Build history of the part. All positions in model axes, mm. Face numbers are marked on the shaded views. A direction names the side the tool comes from. Coordinates: 2 decimals unless noted, no trailing zeros. Loops run counter-clockwise (first coordinate to the right, second up) from the corner with the lowest first, then second, coordinate; pieces in that order, holes last.
Item 1: Cut at D-D (z = 3.5). List the corners of the cut face in (x, y), and give its area (3 significant figures).
Item 2: Cut at C-C (y = 13.5). List the corners of the cut face in (x, z).
Item 3: Flat gauge pins, fed straight in: pin 1 (12 mm diameter, centred on x = 25.5, y = 21.5, fed in from +Z); pin 2 (2.5 mm diameter, centred on y = 41.5, z = 9, fed in from +X); pin 3 (8 mm diameter, centred on y = 2.5, z = 14, fed in from -X). Where does each tip first touch, or does it go through?
Item 4: Cut at A-A (x = 30). List the corners of the cut face in (y, z).
Item 5: Drill centre lines: line 1 along Y through (x, z) = (53.5, 1.3); line 2 along X through (y, z) = (39.15, 12.5); line 3 along X through (y, z) = (34.5, 3.5). Where is each one in solid material? Low to high.
Item 6: Cut at B-B (z = 7). List the corners of the cut face in (x, y), and give its area (3 significant figures).
Item 7: 3-axis set-ups, long thin cutter, end or side, ignore diameter. For the marked faces 1, 2 and 3: which of +Z, -Z, +X, -X, +Y, -Y reach the whole face in a straight line?
Item 8: Mould opens along Y. For the marked faces 4, 5 and 6 say: released by +Y, released by -Y, zero draft, split by the parting line, or undercut.
Autodesk Inventor part; units mm, degrees
ref_plane "YZ Plane" through (0, 0, 0) normal (1, 0, 0) x (0, 1, 0)
ref_plane "XZ Plane" through (0, 0, 0) normal (0, 1, 0) x (-1, 0, 0)
ref_plane "XY Plane" through (0, 0, 0) normal (0, 0, 1) x (1, 0, 0)
sketch "Эскиз1" plane through (0, 0, 0) normal (0, 0, 1) x (1, 0, 0)
  arc A0 (50, 23.4174) -> (30, 23.4174) centre (40, 28) ccw
  line L0 (0, 37.25) -> (5.75, 43)
  line L1 (0, 0) -> (0, 37.25)
  line L2 (80, 0) -> (0, 0)
  line L3 (80, 0) -> (80, 37.25)
  line L4 (74.25, 43) -> (80, 37.25)
  line L5 (5.75, 43) -> (74.25, 43)
  circle A1 centre (40, 28) radius 2
  arc A2 (2.9, 3.4608) -> (7.1, 3.4608) centre (5, 3.4608) ccw
  line L6 (2.9, 3.4608) -> (2.9, 36.5392)
  arc A3 (7.1, 36.5392) -> (2.9, 36.5392) centre (5, 36.5392) ccw
  line L7 (7.1, 36.5392) -> (7.1, 3.4608)
  arc A4 (77.1, 36.5392) -> (72.9, 36.5392) centre (75, 36.5392) ccw
  line L8 (77.1, 36.5392) -> (77.1, 3.4608)
  arc A5 (72.9, 3.4608) -> (77.1, 3.4608) centre (75, 3.4608) ccw
  line L9 (72.9, 3.4608) -> (72.9, 36.5392)
  point P0 (40, -34)
extrude "Выдавливание1" add sketch "Эскиз1" along normal blind 5
sketch "Эскиз2" plane through (0, 0, 5) normal (0, 0, 1) x (1, 0, 0)
  line L0 (60, 0) -> (60, 7.5)
  line L1 (60, 7.5) -> (20, 7.5)
  line L2 (20, 7.5) -> (20, 0)
  line L3 (0, 0) -> (80, 0)
  line L4 (40, 0) -> (60, 7.5) construction
  line L5 (40, 0) -> (20, 7.5) construction
  line L6 (60, 0) -> (20, 0)
  dimension "d2" = 40
extrude "Выдавливание2" add sketch "Эскиз2" along normal blind 15
sketch "Эскиз3" plane through (20, 7.5, 5) normal (0, 1, 0) x (1, 0, 0)
  line L0 (0, 0) -> (0, -15)
  line L1 (0, -7.5) -> (40, -7.5)
  line L2 (40, 0) -> (40, -15)
  line L3 (20, -7.5) -> (20, -15)
  line L4 (20, -7.5) -> (20, 0)
  circle A0 centre (10, -7.5) radius 1.95
  circle A1 centre (30, -7.5) radius 1.95
  point P0 (-20, 5)
  dimension "d6" = 3.9
extrude "Выдавливание3" cut sketch "Эскиз3" against normal blind 15
sketch "Эскиз4" plane through (20, 7.5, 5) normal (0, 1, 0) x (1, 0, 0)
  circle A0 centre (10, -7.5) radius 1.95
  circle A1 centre (10, -7.5) radius 4
  circle A2 centre (30, -7.5) radius 1.95
  circle A3 centre (30, -7.5) radius 4
  point P0 (-20, 5)
  dimension "d9" = 8
  dimension "d10" = 8
extrude "Выдавливание4" cut sketch "Эскиз4" against normal blind 3
sketch "Эскиз5" plane through (0, 0, 0) normal (0, 0, -1) x (-1, 0, 0)
  arc A0 (-30, 23.4174) -> (-50, 23.4174) centre (-40, 28) ccw
  line L0 (-30, 23.4174) -> (-30, 0)
  line L1 (-11.1, 0) -> (-30, 0)
  line L2 (-11.1, 0) -> (-11.1, 37.25)
  line L3 (-13.85, 40) -> (-11.1, 37.25)
  line L4 (-66.15, 40) -> (-13.85, 40)
  line L5 (-68.9, 37.25) -> (-66.15, 40)
  line L6 (-68.9, 0) -> (-68.9, 37.25)
  line L7 (-50, 0) -> (-68.9, 0)
  line L8 (-50, 0) -> (-50, 23.4174)
  circle A1 centre (-26.5, 13.5) radius 1.3
  circle A2 centre (-53.5, 21.5) radius 1.3
  circle A3 centre (-53.5, 5.5) radius 1.3
  circle A4 centre (-53.5, 13.5) radius 1.3
  circle A5 centre (-26.5, 5.5) radius 1.3
  circle A6 centre (-26.5, 21.5) radius 1.3
  circle A7 centre (-40, 28) radius 2
  circle A8 centre (-40, 28) radius 2
  point P0 (0, 0)
  point P1 (28.9, -34)
extrude "Выдавливание5" cut sketch "Эскиз5" against normal through all contours A1 | A2 | A4 | A6
sketch "Эскиз9" plane through (5.75, 43, 0) normal (0, 1, 0) x (1, 0, 0)
  line L0 (54.25, -20) -> (14.25, -20)
  line L1 (14.25, -5) -> (54.25, -5)
  line L2 (54.25, -20) -> (14.25, -20)
  line L3 (14.25, -20) -> (14.25, -5)
  line L4 (14.25, -5) -> (54.25, -5)
  line L5 (54.25, -5) -> (54.25, -20)
  circle A0 centre (44.25, -12.5) radius 1.95
  circle A1 centre (44.25, -12.5) radius 1.95
  circle A2 centre (24.25, -12.5) radius 1.95
  circle A3 centre (24.25, -12.5) radius 1.95
  point P0 (-5.75, 0)
extrude "Выдавливание8" add sketch "Эскиз9" against normal blind 5
properties part number "КВ33.044.702 - Стойка натягивающих роликов оси Y" material "Пластик АБС"
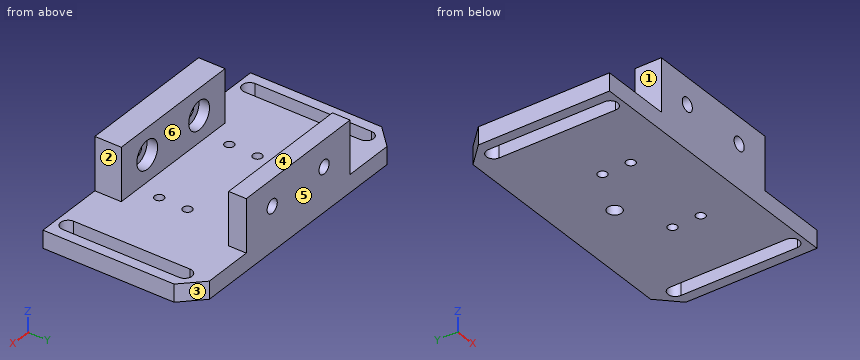
Filled sheet:
1. outline: (0, 0) - (80, 0) - (80, 37.25) - (74.25, 43) - (5.75, 43) - (0, 37.25) - close; hole (2.9, 3.46) arc R2.1 ccw to (7.1, 3.46) - (7.1, 36.54) arc R2.1 ccw to (2.9, 36.54) - close; hole circle Ø2.6 at (26.5, 13.5); hole circle Ø2.6 at (26.5, 21.5); hole circle Ø4 at (40, 28); hole circle Ø2.6 at (53.5, 13.5); hole circle Ø2.6 at (53.5, 21.5); hole (72.9, 3.46) arc R2.1 ccw to (77.1, 3.46) - (77.1, 36.54) arc R2.1 ccw to (72.9, 36.54) - close
1. area: 3,070 mm2
2. outline: (0, 0) - (2.9, 0) - (2.9, 5) - (0, 5) - close; (7.1, 0) - (25.2, 0) - (25.2, 5) - (7.1, 5) - close; (27.8, 0) - (52.2, 0) - (52.2, 5) - (27.8, 5) - close; (54.8, 0) - (72.9, 0) - (72.9, 5) - (54.8, 5) - close; (77.1, 0) - (80, 0) - (80, 5) - (77.1, 5) - close
3. pin 1: stops at z = 5
3. pin 2: stops at x = 60
3. pin 3: stops at x = 20
4. outline: (0, 0) - (43, 0) - (43, 10.55) - (38, 10.55) - (38, 5) - (7.5, 5) - (7.5, 8.5) - (4.5, 8.5) - (4.5, 10.55) - (0, 10.55) - close; (0, 14.45) - (4.5, 14.45) - (4.5, 16.5) - (7.5, 16.5) - (7.5, 20) - (0, 20) - close; (38, 14.45) - (43, 14.45) - (43, 20) - (38, 20) - close
5. line 1: y = 0 to 12.2, 14.8 to 20.2, 22.8 to 43
5. line 2: x = 20 to 28.05, 31.95 to 48.05, 51.95 to 60
5. line 3: x = 0 to 2.9, 7.1 to 72.9, 77.1 to 80
6. outline: (20, 0) - (60, 0) - (60, 7.5) - (20, 7.5) - close; (20, 38) - (60, 38) - (60, 43) - (20, 43) - close
6. area: 500 mm2
7. face 1: +Z, -X, +Y, -Y
7. face 2: +Z, +X, +Y, -Y
7. face 3: +Z, -Z, +X, +Y
8. face 4: zero draft
8. face 5: released by +Y
8. face 6: undercut
